Geometry: see drawing. Coordinates: mm, zero at the bounding-box minimum. A direction names the side the tool comes from. Coordinates: 2 decimals unless noted, no trailing zeros. Loops run counter-clockwise (first coordinate to the right, second up) from the corner with the lowest first, then second, coordinate; pieces in that order, holes last. Notation, with made-up numbers: M -26.5,64.25 L -5.5,64.25 A21 ccw -5.5,78.25 Z; hole C 35.5,-24.75 d7. An arc over 180 degrees is marked long. One line per question, with ' | ' between items. Start each with the question number.
1. Mould query, pull axis X, two halves, no side actions, for the marked faces 3, 4 and 5. Classes: pulls with the +X half, pulls with the -X half, needs draft (parallel to the pull), parting line crosses it, or undercut.
2. Section query D-D, the plane y = 1.5. Output: boundary loops of the cut face in (x, z).
3. Section query B-B, the plane z = 6. Output: boundary loops of the cut face in (x, y).
4. Pin query (flat end, axial travel): P1, Ø2, axis at x = 3.5, y = 2, coming from the -Z side. Return the tip coordinate at first contact, or that it passes through.
5. Section query A-A, the plane x = 6. Output: boundary loops of the cut face in (y, z).
6. Ray query, probe 1 along X at (y, z) = (1.6, 6); probe 2 along Y at (x, z) = (3, 1); probe 3 along Z at (x, y) = (6, 1.25). Return the intervals inside material, ascending.
7. Access query for the marked faces 1 and 2. Directions: +Z, -Z, +X, -X, +Y, -Y. A direction counts if a zero-diameter tool reaches every point of the face in a straight line with its end or side. Return the directions, or none.
8. Section query C-C, the plane y = 0.5. Output: boundary loops of the cut face in (x, z).
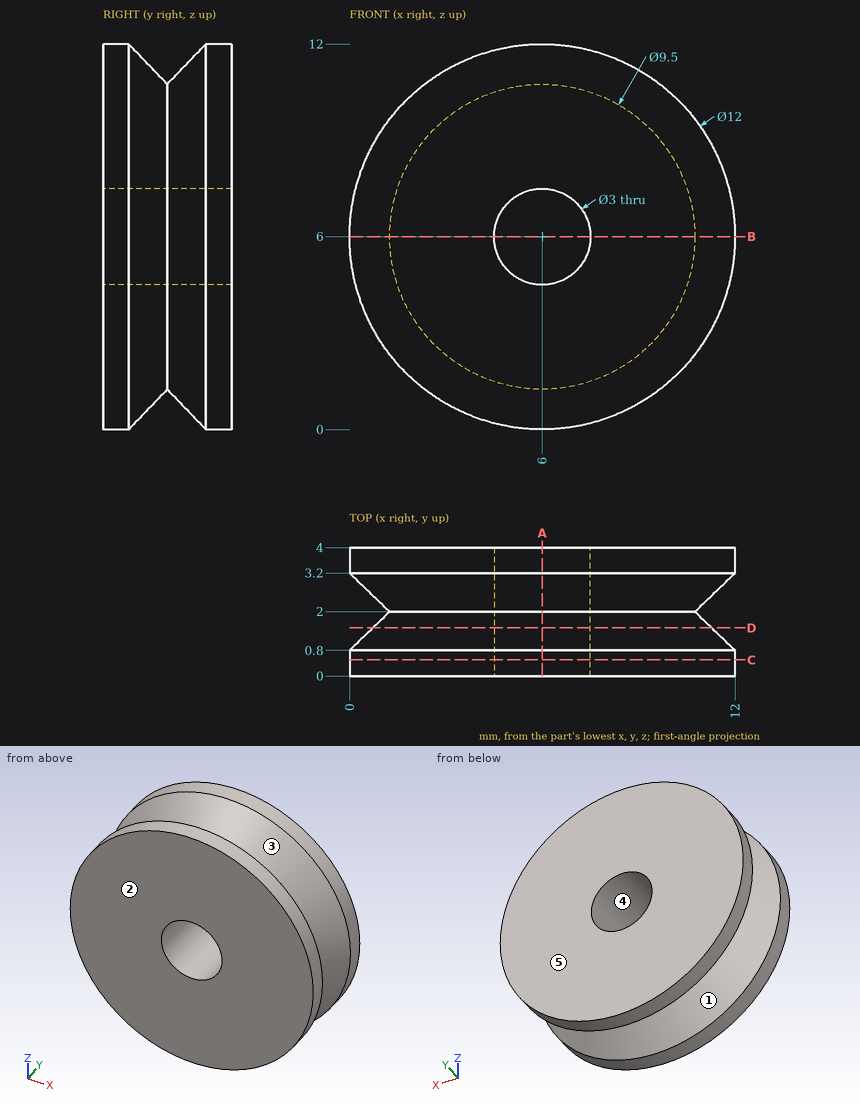
Taken from the geometry:
1) face 3: parting line crosses it | face 4: undercut | face 5: needs draft
2) outline: C 6,6 d10.54; hole C 6,6 d3
3) outline: M 0,0 L 4.5,0 L 4.5,4 L 0,4 L 0,3.2 L 1.25,2 L 0,0.8 Z; M 7.5,0 L 12,0 L 12,0.8 L 10.75,2 L 12,3.2 L 12,4 L 7.5,4 Z
4) P1: z = 0.69
5) outline: M 0,0 L 0.8,0 L 2,1.25 L 3.2,0 L 4,0 L 4,4.5 L 0,4.5 Z; M 0,7.5 L 4,7.5 L 4,12 L 3.2,12 L 2,10.75 L 0.8,12 L 0,12 Z
6) probe 1: 0.83 to 4.5, 7.5 to 11.17 | probe 2: 0 to 0.96, 3.04 to 4 | probe 3: 0.47 to 4.5, 7.5 to 11.53
7) face 1: none | face 2: +Z, -Z, +X, -X, -Y
8) outline: C 6,6 d12; hole C 6,6 d3
